from build123d import *

# Parameters (mm, degrees)
SZKIC1_R                    = 1.55
SZKIC1_R_2                  = 1.6
DODANIE_WYCI_GNI_CIE1_DEPTH = 8
ZAOKR_GLENIE1_R             = 4
SZKIC2_R                    = 3
WYTNIJ_WYCI_GNI_CIE1_DEPTH  = 3
ZAOKR_GLENIE2_R             = 1
SFAZOWANIE1_SIZE            = 0.25
WYTNIJ_WYCI_GNI_CIE2_DEPTH  = 1


with BuildPart() as part:
    # Szkic1 → Dodanie-wyciągnięcie1 (new body)
    with BuildSketch(Plane.XY):
        Polygon((-32.374614688, -34.065144123), (1.443331859, 8.207289062), (26.5780588, -66), (-24.095207609, -66), align=None)
        with Locations((-21, -62)):
            Circle(SZKIC1_R, mode=Mode.SUBTRACT)
        with Locations((21, -62)):
            Circle(SZKIC1_R, mode=Mode.SUBTRACT)
        Circle(SZKIC1_R_2, mode=Mode.SUBTRACT)
        with Locations((-28, -35)):
            Circle(SZKIC1_R_2, mode=Mode.SUBTRACT)
        Polygon((-23.625385312, -35.934855877), (-1.443331859, -8.207289062), (15.4219412, -58), (-17.904792391, -58), align=None, mode=Mode.SUBTRACT)
    extrude(amount=DODANIE_WYCI_GNI_CIE1_DEPTH)

    # Zaokrąglenie1
    zaokr_glenie1_edges = [part.edges().sort_by_distance(p)[0] for p in [
        (-32.374614688, -34.065144123, 4),
        (1.443331859, 8.207289062, 4),
        (26.5780588, -66, 4),
        (-24.095207609, -66, 4),
    ]]
    fillet(zaokr_glenie1_edges, radius=ZAOKR_GLENIE1_R)

    # Szkic2 → Wytnij-wyciągnięcie1 (cut)
    with BuildSketch(Plane.XY.offset(8)):
        Circle(SZKIC2_R)
        with Locations((-28, -35)):
            Circle(SZKIC2_R)
        with Locations((-21, -62)):
            Circle(SZKIC2_R)
        with Locations((21, -62)):
            Circle(SZKIC2_R)
    extrude(amount=-WYTNIJ_WYCI_GNI_CIE1_DEPTH, mode=Mode.SUBTRACT)

    # Zaokrąglenie2
    zaokr_glenie2_edges = [part.edges().sort_by_distance(p)[0] for p in [
        (-23.625385312, -35.934855877, 4),
        (-17.904792391, -58, 4),
        (15.4219412, -58, 4),
        (-1.443331859, -8.207289062, 4),
    ]]
    fillet(zaokr_glenie2_edges, radius=ZAOKR_GLENIE2_R)

    # Sfazowanie1
    sfazowanie1_edges = [part.edges().sort_by_distance(p)[0] for p in [
        (7.058775414, -33.30874863, 0),
        (7.058775414, -33.30874863, 8),
        (-20.799357962, -46.835247082, 0),
        (-20.799357962, -46.835247082, 8),
        (-12.948817041, -22.589145539, 0),
        (-12.948817041, -22.589145539, 8),
        (14.84007865, -57.582749074, 0),
        (14.84007865, -57.582749074, 8),
        (-17.742969998, -57.790873618, 0),
        (-17.742969998, -57.790873618, 8),
        (-23.509651218, -35.959588272, 0),
        (-23.509651218, -35.959588272, 8),
        (-1.630962951, -9.274224983, 0),
        (-1.630962951, -9.274224983, 8),
        (0, -66, 0),
        (0, -66, 8),
        (-28.371987593, -49.503848635, 0),
        (-17.123475238, -15.00121981, 0),
        (14.288578303, -29.716771865, 0),
        (0.692807492, 3.939545377, 0),
        (24.2506086, -64.330996296, 0),
        (-31.911678313, -34.164073702, 0),
        (-23.44791804, -65.163494471, 0),
        (-28.371987593, -49.503848635, 8),
        (14.288578303, -29.716771865, 8),
        (-17.123475238, -15.00121981, 8),
        (0.692807492, 3.939545377, 8),
        (24.2506086, -64.330996296, 8),
        (-31.911678313, -34.164073702, 8),
        (-23.44791804, -65.163494471, 8),
        (-3, 0, 8),
        (-31, -35, 8),
        (-24, -62, 8),
        (18, -62, 8),
        (-1.551781994, -58, 0),
        (-1.551781994, -58, 8),
    ]]
    chamfer(sfazowanie1_edges, length=SFAZOWANIE1_SIZE)

    # Szkic3 → Wytnij-wyciągnięcie2 (cut)
    with BuildSketch(Plane(origin=(0, 0, 0), x_dir=(-1, 0, 0), z_dir=(0, 0, -1))):
        Polygon((-11, -60.5), (-11, -63.5), (-7.291900756, -62), align=None)
    extrude(amount=-WYTNIJ_WYCI_GNI_CIE2_DEPTH, mode=Mode.SUBTRACT)


solid = part.part
Check sheet for the modelled part. Datum: model origin and axes. Units: mm. A direction names the side the tool comes from. Round coordinates to 2 decimals unless told otherwise and drop trailing zeros. Loops run counter-clockwise (first coordinate to the right, second up) from the corner with the lowest first, then second, coordinate; pieces in that order, holes last. Notation, with made-up numbers: M -25.75,59 L 26.25,59 A37 ccw 26.25,96 Z; hole C 44,-37.75 d2. An arc over 180 degrees is marked long. One line per question, with ' | ' between items. Start each with the question number.
Item 1: Scan lines: probe 1 along X at (y, z) = (-62, 3.5); probe 2 along X at (y, z) = (-52, 2.5); probe 3 along X at (y, z) = (-35, 3). Record each from-to range of solid material in increasing order.
Item 2: Set-up check for faces 1 (the face through (6.948, -32.982, 3.948)), 2 (the face through (7.06, -32.94, 0.13)), 3 (the face through (24.28, -64.29, 4.05)), 4 (the face through (-28.204, -49.662, 0.127)), 5 (the face through (-19.7, -63.3, 5)): record each of +Z, -Z, +X, -X, +Y, -Y from which the full face is reachable in a straight line by a thin tool's end or side.
Item 3: Section check A-A (y = 0). Record the boundary of the cut face in (x, z).
Item 4: Section check B-B (z = 1.75). Record the boundary of the cut face in (x, y), and give its area (3 significant figures).
Item 5: Section check D-D (x = 0.5). State how many separate pieces and enclosed holes the cut face has, and give its area (3 significant figures).
Item 6: Gauge pin test, flat ends, axial feed: pin 1 Ø3 at (y, z) = (-16, 6.5) entering from +X; pin 2 Ø2 at (x, z) = (-25.5, 2) entering from +Y; pin 3 Ø1.8 at (x, y) = (20, -62) entering from +Z. Record the tip position at first contact, or that the pin passes through.
Item 7: Section check C-C (x = -7). Record the boundary of the cut face in (y, z).
Worked out:
1) probe 1: -25.13 to -22.55, -19.45 to 19.45, 22.55 to 25 | probe 2: -27.72 to -19.46, 13.39 to 21.84 | probe 3: -32 to -29.6, -26.4 to -22.88, 7.63 to 16.08
2) face 1: +Z, -Z | face 2: -Z | face 3: +Z, -Z, +X | face 4: -Z, -X, -Y | face 5: +Z
3) outline: M -5.12,0.25 L -4.8,0 L -1.6,0 L -1.6,5 L -3,5 L -3,7.75 L -3.25,8 L -4.8,8 L -5.12,7.75 Z; M 1.6,0 L 3.96,0 L 4.22,0.25 L 4.22,7.75 L 3.96,8 L 3.25,8 L 3,7.75 L 3,5 L 1.6,5 Z
4) outline: M -31.87,-36 L -24.87,-63 A4 ccw -21,-66 L 21,-66 A4 ccw 24.79,-60.72 L 3.79,1.28 A4 ccw -3.12,2.5 L -31.12,-32.5 A4 ccw Z; hole C -28,-35 d3.2; hole M -23.5,-36.42 L -18.1,-57.25 A1 ccw -17.13,-58 L 14.03,-58 A1 ccw 14.97,-56.68 L -0.86,-9.94 A1 ccw -2.59,-9.63 L -23.31,-35.54 A1 ccw Z; hole C -21,-62 d3.1; hole C 0,0 d3.2; hole C 21,-62 d3.1 | area: 1,390 mm^2
5) separate pieces: 3 | enclosed holes: 0 | area: 174 mm^2
6) pin 1: x = 10.15 | pin 2: y = -24.22 | pin 3: z = 5
7) outline: M -66,0.25 L -65.75,0 L -58.25,0 L -58,0.25 L -58,7.75 L -58.25,8 L -65.75,8 L -66,7.75 Z; M -15.15,0.25 L -14.75,0 L -2.75,0 L -2.35,0.25 L -2.35,7.75 L -2.75,8 L -14.75,8 L -15.15,7.75 Z
